The model under review builds one solid part; all positions refer to its coordinate system, in mm. Give positions to 0.01 mm unless a question says otherwise; leave off trailing zeros. Order: outer loops, then holes, each group sorted by start corner. A loop starts at its lowest first (then second) coordinate and runs counter-clockwise, first axis right, second up. Notation, with made-up numbers: (85, 9) -> (103, 9) arc R13 ccw to (103, 31) -> close; hole circle Ø7 at (-25, -22.75). An arc over 180 degrees is marked (long way). Answer as a JSON object with one key per item and string values. Group by question number.
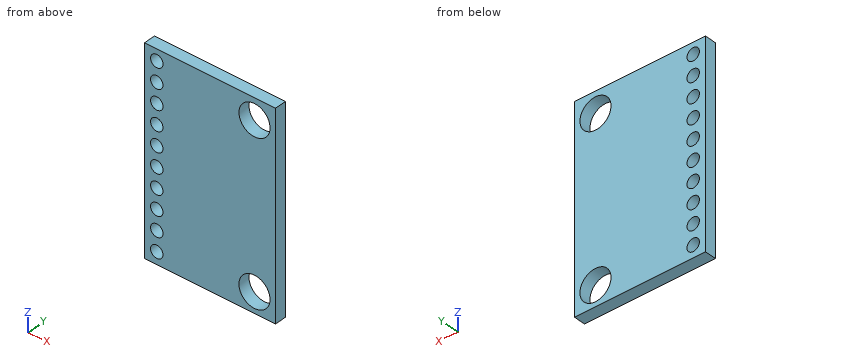
from build123d import *

# Parameters (mm, degrees)
SKETCH1_W           = 16.86
SKETCH1_H           = 25.88
BOSS_EXTRUDE1_DEPTH = 1.5
CUT_EXTRUDE1_REACH  = 3.5
SKETCH2_R           = 2
CUT_EXTRUDE2_REACH  = 3.5
SKETCH3_R           = 0.8


with BuildPart() as part:
    # Sketch1 → Boss-Extrude1 (new body)
    with BuildSketch(Plane(origin=(0, 0, 0), x_dir=(1, 0, 0), z_dir=(0, 1, 0))):
        with Locations((8.43, 12.94)):
            Rectangle(SKETCH1_W, SKETCH1_H)
    extrude(amount=BOSS_EXTRUDE1_DEPTH)

    # Sketch2 → Cut-Extrude1 (cut, up to next)
    with BuildSketch(Plane(origin=(0, 1.5, 0), x_dir=(1, 0, 0), z_dir=(0, 1, 0)), mode=Mode.PRIVATE) as cut_extrude1_sk1:
        with Locations((14.16, 23.28)):
            Circle(SKETCH2_R)
    cut_extrude1_tool1 = extrude(cut_extrude1_sk1.sketch, amount=-CUT_EXTRUDE1_REACH, mode=Mode.PRIVATE) & part.part
    add(cut_extrude1_tool1.solids().sort_by_distance((14.16, 1.5, -23.28))[0], mode=Mode.SUBTRACT)
    # Sketch2 → Cut-Extrude1 (cut, up to next)
    with BuildSketch(Plane(origin=(0, 1.5, 0), x_dir=(1, 0, 0), z_dir=(0, 1, 0)), mode=Mode.PRIVATE) as cut_extrude1_sk2:
        with Locations((14.16, 2.7)):
            Circle(SKETCH2_R)
    cut_extrude1_tool2 = extrude(cut_extrude1_sk2.sketch, amount=-CUT_EXTRUDE1_REACH, mode=Mode.PRIVATE) & part.part
    add(cut_extrude1_tool2.solids().sort_by_distance((14.16, 1.5, -2.7))[0], mode=Mode.SUBTRACT)

    # Sketch3 → Cut-Extrude2 (cut, up to next)
    with BuildSketch(Plane(origin=(0, 1.5, 0), x_dir=(1, 0, 0), z_dir=(0, 1, 0)), mode=Mode.PRIVATE) as cut_extrude2_sk1:
        with Locations((1.58, 24.32)):
            Circle(SKETCH3_R)
    cut_extrude2_tool1 = extrude(cut_extrude2_sk1.sketch, amount=-CUT_EXTRUDE2_REACH, mode=Mode.PRIVATE) & part.part
    add(cut_extrude2_tool1.solids().sort_by_distance((1.58, 1.5, -24.32))[0], mode=Mode.SUBTRACT)
    # Sketch3 → Cut-Extrude2 (cut, up to next)
    with BuildSketch(Plane(origin=(0, 1.5, 0), x_dir=(1, 0, 0), z_dir=(0, 1, 0)), mode=Mode.PRIVATE) as cut_extrude2_sk2:
        with Locations((1.58, 21.78)):
            Circle(SKETCH3_R)
    cut_extrude2_tool2 = extrude(cut_extrude2_sk2.sketch, amount=-CUT_EXTRUDE2_REACH, mode=Mode.PRIVATE) & part.part
    add(cut_extrude2_tool2.solids().sort_by_distance((1.58, 1.5, -21.78))[0], mode=Mode.SUBTRACT)
    # Sketch3 → Cut-Extrude2 (cut, up to next)
    with BuildSketch(Plane(origin=(0, 1.5, 0), x_dir=(1, 0, 0), z_dir=(0, 1, 0)), mode=Mode.PRIVATE) as cut_extrude2_sk3:
        with Locations((1.58, 19.24)):
            Circle(SKETCH3_R)
    cut_extrude2_tool3 = extrude(cut_extrude2_sk3.sketch, amount=-CUT_EXTRUDE2_REACH, mode=Mode.PRIVATE) & part.part
    add(cut_extrude2_tool3.solids().sort_by_distance((1.58, 1.5, -19.24))[0], mode=Mode.SUBTRACT)
    # Sketch3 → Cut-Extrude2 (cut, up to next)
    with BuildSketch(Plane(origin=(0, 1.5, 0), x_dir=(1, 0, 0), z_dir=(0, 1, 0)), mode=Mode.PRIVATE) as cut_extrude2_sk4:
        with Locations((1.58, 16.7)):
            Circle(SKETCH3_R)
    cut_extrude2_tool4 = extrude(cut_extrude2_sk4.sketch, amount=-CUT_EXTRUDE2_REACH, mode=Mode.PRIVATE) & part.part
    add(cut_extrude2_tool4.solids().sort_by_distance((1.58, 1.5, -16.7))[0], mode=Mode.SUBTRACT)
    # Sketch3 → Cut-Extrude2 (cut, up to next)
    with BuildSketch(Plane(origin=(0, 1.5, 0), x_dir=(1, 0, 0), z_dir=(0, 1, 0)), mode=Mode.PRIVATE) as cut_extrude2_sk5:
        with Locations((1.58, 14.16)):
            Circle(SKETCH3_R)
    cut_extrude2_tool5 = extrude(cut_extrude2_sk5.sketch, amount=-CUT_EXTRUDE2_REACH, mode=Mode.PRIVATE) & part.part
    add(cut_extrude2_tool5.solids().sort_by_distance((1.58, 1.5, -14.16))[0], mode=Mode.SUBTRACT)
    # Sketch3 → Cut-Extrude2 (cut, up to next)
    with BuildSketch(Plane(origin=(0, 1.5, 0), x_dir=(1, 0, 0), z_dir=(0, 1, 0)), mode=Mode.PRIVATE) as cut_extrude2_sk6:
        with Locations((1.58, 11.62)):
            Circle(SKETCH3_R)
    cut_extrude2_tool6 = extrude(cut_extrude2_sk6.sketch, amount=-CUT_EXTRUDE2_REACH, mode=Mode.PRIVATE) & part.part
    add(cut_extrude2_tool6.solids().sort_by_distance((1.58, 1.5, -11.62))[0], mode=Mode.SUBTRACT)
    # Sketch3 → Cut-Extrude2 (cut, up to next)
    with BuildSketch(Plane(origin=(0, 1.5, 0), x_dir=(1, 0, 0), z_dir=(0, 1, 0)), mode=Mode.PRIVATE) as cut_extrude2_sk7:
        with Locations((1.58, 9.08)):
            Circle(SKETCH3_R)
    cut_extrude2_tool7 = extrude(cut_extrude2_sk7.sketch, amount=-CUT_EXTRUDE2_REACH, mode=Mode.PRIVATE) & part.part
    add(cut_extrude2_tool7.solids().sort_by_distance((1.58, 1.5, -9.08))[0], mode=Mode.SUBTRACT)
    # Sketch3 → Cut-Extrude2 (cut, up to next)
    with BuildSketch(Plane(origin=(0, 1.5, 0), x_dir=(1, 0, 0), z_dir=(0, 1, 0)), mode=Mode.PRIVATE) as cut_extrude2_sk8:
        with Locations((1.58, 6.54)):
            Circle(SKETCH3_R)
    cut_extrude2_tool8 = extrude(cut_extrude2_sk8.sketch, amount=-CUT_EXTRUDE2_REACH, mode=Mode.PRIVATE) & part.part
    add(cut_extrude2_tool8.solids().sort_by_distance((1.58, 1.5, -6.54))[0], mode=Mode.SUBTRACT)
    # Sketch3 → Cut-Extrude2 (cut, up to next)
    with BuildSketch(Plane(origin=(0, 1.5, 0), x_dir=(1, 0, 0), z_dir=(0, 1, 0)), mode=Mode.PRIVATE) as cut_extrude2_sk9:
        with Locations((1.58, 4)):
            Circle(SKETCH3_R)
    cut_extrude2_tool9 = extrude(cut_extrude2_sk9.sketch, amount=-CUT_EXTRUDE2_REACH, mode=Mode.PRIVATE) & part.part
    add(cut_extrude2_tool9.solids().sort_by_distance((1.58, 1.5, -4))[0], mode=Mode.SUBTRACT)
    # Sketch3 → Cut-Extrude2 (cut, up to next)
    with BuildSketch(Plane(origin=(0, 1.5, 0), x_dir=(1, 0, 0), z_dir=(0, 1, 0)), mode=Mode.PRIVATE) as cut_extrude2_sk10:
        with Locations((1.58, 1.46)):
            Circle(SKETCH3_R)
    cut_extrude2_tool10 = extrude(cut_extrude2_sk10.sketch, amount=-CUT_EXTRUDE2_REACH, mode=Mode.PRIVATE) & part.part
    add(cut_extrude2_tool10.solids().sort_by_distance((1.58, 1.5, -1.46))[0], mode=Mode.SUBTRACT)


solid = part.part
1. For probe 1 along Z at (x, y) = (14.16, 0.35); probe 2 along X at (y, z) = (0.3, -23.75); probe 3 along X at (y, z) = (0.85, -19.24), list the stretches that pass through material, from the lowest coordinate up. Write a range as [from, to].
2. Take a section at B-B on y = 0.65. State how many separate pieces and enclosed holes the cut face has, plus the area to 3 significant figures.
3. Take a section at C-C on x = 14.16. Give the boundary of the cut face in (y, z).
4. Take a section at D-D on z = -2.7. Give the boundary of the cut face in (x, y), plus the area to 3 significant figures.
5. Take a section at A-A on z = -14.16. Give the boundary of the cut face in (x, y).
Checks:
{
 "1": {"probe 1": "z = [-25.88, -25.28], [-21.28, -4.7], [-0.7, 0]", "probe 2": "x = [0, 1.02], [2.14, 12.22], [16.1, 16.86]", "probe 3": "x = [0, 0.78], [2.38, 16.86]"},
 "2": {"separate pieces": "1", "enclosed holes": "12", "area": "391 mm2"},
 "3": {"outline": "(0, -25.88) -> (1.5, -25.88) -> (1.5, -25.28) -> (0, -25.28) -> close; (0, -21.28) -> (1.5, -21.28) -> (1.5, -4.7) -> (0, -4.7) -> close; (0, -0.7) -> (1.5, -0.7) -> (1.5, 0) -> (0, 0) -> close"},
 "4": {"outline": "(0, 0) -> (12.16, 0) -> (12.16, 1.5) -> (0, 1.5) -> close; (16.16, 0) -> (16.86, 0) -> (16.86, 1.5) -> (16.16, 1.5) -> close", "area": "19.3 mm2"},
 "5": {"outline": "(0, 0) -> (0.78, 0) -> (0.78, 1.5) -> (0, 1.5) -> close; (2.38, 0) -> (16.86, 0) -> (16.86, 1.5) -> (2.38, 1.5) -> close"}
}
